Part model, mm, in its own coordinate system. Round coordinates to 2 decimals unless told otherwise and drop trailing zeros. Loops run counter-clockwise (first coordinate to the right, second up) from the corner with the lowest first, then second, coordinate; pieces in that order, holes last.
Autodesk Inventor part; units mm, degrees
ref_plane "YZ Plane" through (0, 0, 0) normal (1, 0, 0) x (0, 1, 0)
ref_plane "XZ Plane" through (0, 0, 0) normal (0, 1, 0) x (-1, 0, 0)
ref_plane "XY Plane" through (0, 0, 0) normal (0, 0, 1) x (1, 0, 0)
sketch "Sketch1" plane through (0, 0, 0) normal (0, 0, 1) x (1, 0, 0)
  line L0 (0, 0) -> (101.6, 0)
  line L1 (101.6, 0) -> (101.6, 63.5)
  line L2 (101.6, 63.5) -> (0, 63.5)
  line L3 (0, 63.5) -> (0, 0)
  line L4 (7.1778, 63.5) -> (7.1778, 57.15)
  line L5 (0, 57.15) -> (6.35, 57.15)
  line L6 (6.35, 57.15) -> (44.45, 57.15)
  line L7 (44.45, 57.15) -> (95.25, 57.15)
  circle A0 centre (44.45, 57.15) radius 2.54
  circle A1 centre (95.25, 57.15) radius 2.54
  circle A2 centre (6.35, 57.15) radius 2.54
  line L8 (6.35, 0) -> (6.35, 6.35)
  line L9 (0, 6.35) -> (6.35, 6.35)
  line L10 (6.35, 6.35) -> (44.45, 6.35)
  line L11 (44.45, 6.35) -> (69.85, 6.35)
  line L12 (69.85, 6.35) -> (95.25, 6.35)
  circle A3 centre (6.35, 6.35) radius 2.54
  circle A4 centre (44.45, 6.35) radius 2.54
  circle A5 centre (95.25, 6.35) radius 2.54
  dimension "d0" = 101.6
  dimension "d1" = 63.5
  dimension "d2" = 6.35
  dimension "d3" = 6.35
  dimension "d5" = 38.1
  dimension "d6" = 50.8
  dimension "d7" = 5.08
  dimension "d8" = 5.08
  dimension "d9" = 5.08
  dimension "d12" = 6.35
  dimension "d13" = 6.35
  dimension "d14" = 38.1
  dimension "d15" = 25.4
  dimension "d16" = 25.4
  dimension "d17" = 5.08
  dimension "d18" = 5.08
  dimension "d19" = 5.08
extrude "Extrusion1" add sketch "Sketch1" along normal blind 1.5875 contours L3 L9 A3 L8 L0 | L8 A3 L9 L3 L5 A2 L4 L2 L1 L0 | L3 L2 L4 A2 L5
properties part number "kickPlate"
1) Slice it at C-C, the plane z = 0.8. Give the cut face in (x, y), then the cut area to 3 significant figures.
Values:
outline: (0, 0) - (101.6, 0) - (101.6, 63.5) - (0, 63.5) - close; hole circle Ø5.08 at (6.35, 6.35); hole circle Ø5.08 at (6.35, 57.15); hole circle Ø5.08 at (44.45, 6.35); hole circle Ø5.08 at (44.45, 57.15); hole circle Ø5.08 at (95.25, 6.35); hole circle Ø5.08 at (95.25, 57.15)
area: 6,330 mm2
2) Slice it at B-B, the plane x = 6.35. Give the cut face in (y, z), then the cut area to 3 significant figures.
Values:
outline: (0, 0) - (3.81, 0) - (3.81, 1.59) - (0, 1.59) - close; (8.89, 0) - (54.61, 0) - (54.61, 1.59) - (8.89, 1.59) - close; (59.69, 0) - (63.5, 0) - (63.5, 1.59) - (59.69, 1.59) - close
area: 84.7 mm2
3) Mould opens along X. For faces 1 (the face through (50, 32, 1.588)), 2 (the face through (5.8, 8.83, 0.78)) say: released by +X, released by -X, zero draft, split by the parting line, or undercut.
Values:
face 1: zero draft
face 2: undercut
4) Slice it at A-A, the plane y = 6.35. Give the cut face in (x, z).
Values:
outline: (0, 0) - (3.81, 0) - (3.81, 1.59) - (0, 1.59) - close; (8.89, 0) - (41.91, 0) - (41.91, 1.59) - (8.89, 1.59) - close; (46.99, 0) - (92.71, 0) - (92.71, 1.59) - (46.99, 1.59) - close; (97.79, 0) - (101.6, 0) - (101.6, 1.59) - (97.79, 1.59) - close
5) Drop flat-ended pins along their axis: pin 1 Ø6 at (x, y) = (95.25, 6.35) entering from -Z; pin 2 Ø3 at (x, y) = (44.45, 6.35) entering from +Z. Give the stop position or say it passes through.
Values:
pin 1: stops at z = 0
pin 2: passes through
6) Wall check: line 1 along Y through (x, z) = (44.45, 1.15); line 2 along X through (y, z) = (7, 1.4); line 3 along Y through (x, z) = (5, 0.25). Give the ranges that are in metal, low to high.
Values:
line 1: y = 0 to 3.81, 8.89 to 54.61, 59.69 to 63.5
line 2: x = 0 to 3.89, 8.81 to 41.99, 46.91 to 92.79, 97.71 to 101.6
line 3: y = 0 to 4.2, 8.5 to 55, 59.3 to 63.5
